Input: part model. Units: mm. Frame: model coordinates. A direction names the side the tool comes from. Coordinates: 2 decimals unless noted, no trailing zeros. Write each loop counter-clockwise with the first axis right and the second up, starting at its lowest first coordinate (ties: lowest second). Pieces come first, ordered by that corner, then holes. Notation, with made-up numbers: (29, 77.25) - (80, 77.25) arc R22 cw to (80, 114.25) - close; hole circle Ø7 at (73, 42.25). An arc over 180 degrees is marked (long way). Use a Markdown table: item, result. Add a question column.
Q1. Section query B-B (z = 0). Return the cut outline in (x, y).
Q2. Set-up query: faces 5 (the face through (44.99, 2.94, -26.08)), 6 (the face through (-25, 2.3, 8)). Return all of +Z, -Z, +X, -X, +Y, -Y with unobstructed straight access to the full face (end or side cutting, diameter ignored); none if empty.
Q3. Pin query (flat end, axial travel): P1, Ø5, axis at x = 0, z = 54, coming from the +Y side. Return the tip coordinate at first contact, or that it passes through.
Q4. Mould query, pull axis Z, two halves, no side actions, for faces 1 (the face through (2.64, 2.86, -59.94)), 2 (the face through (-19.524, 2.859, -4.336)), 3 (the face through (0, 3, -56)), 4 (the face through (-39, 5.8, -1)). Classes: released by +Z, released by -Z, zero draft, split by the parting line, or undercut.
Q5. Section query D-D (x = 18.5). Return the cut outline in (y, z), then the cut area to 3 significant figures.
Q6. Section query A-A (x = 0). Return the cut outline in (y, z), then the cut area to 3 significant figures.
Q7. Material intervals for probe 1 along X at (y, z) = (4.5, 27); probe 2 along X at (y, z) = (1.65, 27.5); probe 3 along X at (y, z) = (3.3, -9), sorted ascending. Write a range as from..to.
Q8. Section query C-C (y = 3.6). Give the number of separate pieces and of enclosed holes in the cut face, then the cut area to 3 significant figures.
from build123d import *

# Parameters (mm, degrees)
SKETCH1_R           = 60
SKETCH1_R_2         = 20
BOSS_EXTRUDE1_DEPTH = 5.8
SKETCH2_R           = 38.5
SKETCH2_R_2         = 25
CUT_EXTRUDE1_DEPTH  = 3.5
SKETCH3_R           = 2
CUT_EXTRUDE2_DEPTH  = 86.050808344


with BuildPart() as part:
    # Sketch1 → Boss-Extrude1 (new body)
    with BuildSketch(Plane(origin=(0, 0, 0), x_dir=(1, 0, 0), z_dir=(0, 1, 0))):
        with Locations(Location((0, 0, 0), (0, 0, 270))):
            Circle(SKETCH1_R)
        with Locations(Location((0, 0, 0), (0, 0, 270))):
            Circle(SKETCH1_R_2, mode=Mode.SUBTRACT)
    extrude(amount=BOSS_EXTRUDE1_DEPTH)

    # Sketch2 → Cut-Extrude1 (cut)
    with BuildSketch(Plane(origin=(0, 5.8, 0), x_dir=(1, 0, 0), z_dir=(0, 1, 0))):
        with Locations(Location((0, 0, 0), (0, 0, 270))):
            Circle(SKETCH2_R)
        with Locations(Location((0, 0, 0), (0, 0, 270))):
            Circle(SKETCH2_R_2, mode=Mode.SUBTRACT)
    extrude(amount=-CUT_EXTRUDE1_DEPTH, mode=Mode.SUBTRACT)

    # Sketch3 → Cut-Extrude2 (cut, through all)
    with BuildSketch(Plane(origin=(0, 5.8, 0), x_dir=(1, 0, 0), z_dir=(0, 1, 0))):
        with Locations(Location((0, 54, 0), (0, 0, 270))):
            Circle(SKETCH3_R)
        with Locations(Location((46.765371804, 27, 0), (0, 0, 270))):
            Circle(SKETCH3_R)
        with Locations(Location((46.765371804, -27, 0), (0, 0, 270))):
            Circle(SKETCH3_R)
        with Locations(Location((0, -54, 0), (0, 0, 270))):
            Circle(SKETCH3_R)
        with Locations(Location((-46.765371804, -27, 0), (0, 0, 270))):
            Circle(SKETCH3_R)
        with Locations(Location((-46.765371804, 27, 0), (0, 0, 270))):
            Circle(SKETCH3_R)
    extrude(amount=-CUT_EXTRUDE2_DEPTH, mode=Mode.SUBTRACT)


solid = part.part
Values follow:
| question | item | result |
|---|---|---|
| 1 | outline | (-60, 0) - (-20, 0) - (-20, 5.8) - (-25, 5.8) - (-25, 2.3) - (-38.5, 2.3) - (-38.5, 5.8) - (-60, 5.8) - close; (20, 0) - (60, 0) - (60, 5.8) - (38.5, 5.8) - (38.5, 2.3) - (25, 2.3) - (25, 5.8) - (20, 5.8) - close |
| 2 | face 5 | +Y, -Y |
| 2 | face 6 | +Y |
| 3 | P1 | y = 5.8 |
| 4 | face 1 | split by the parting line |
| 4 | face 2 | undercut |
| 4 | face 3 | undercut |
| 4 | face 4 | zero draft |
| 5 | outline | (0, -57.08) - (5.8, -57.08) - (5.8, -33.76) - (2.3, -33.76) - (2.3, -16.82) - (5.8, -16.82) - (5.8, -7.6) - (0, -7.6) - close; (0, 7.6) - (5.8, 7.6) - (5.8, 16.82) - (2.3, 16.82) - (2.3, 33.76) - (5.8, 33.76) - (5.8, 57.08) - (0, 57.08) - close |
| 5 | area | 455 mm2 |
| 6 | outline | (0, -60) - (5.8, -60) - (5.8, -56) - (0, -56) - close; (0, -52) - (5.8, -52) - (5.8, -38.5) - (2.3, -38.5) - (2.3, -25) - (5.8, -25) - (5.8, -20) - (0, -20) - close; (0, 20) - (5.8, 20) - (5.8, 25) - (2.3, 25) - (2.3, 38.5) - (5.8, 38.5) - (5.8, 52) - (0, 52) - close; (0, 56) - (5.8, 56) - (5.8, 60) - (0, 60) - close |
| 6 | area | 323 mm2 |
| 7 | probe 1 | -53.58..-48.77, -44.77..-27.45, 27.45..44.77, 48.77..53.58 |
| 7 | probe 2 | -53.33..-48.7, -44.83..44.83, 48.7..53.33 |
| 7 | probe 3 | -59.32..-37.43, -23.32..-17.86, 17.86..23.32, 37.43..59.32 |
| 8 | separate pieces | 2 |
| 8 | enclosed holes | 8 |
| 8 | area | 7,280 mm2 |
